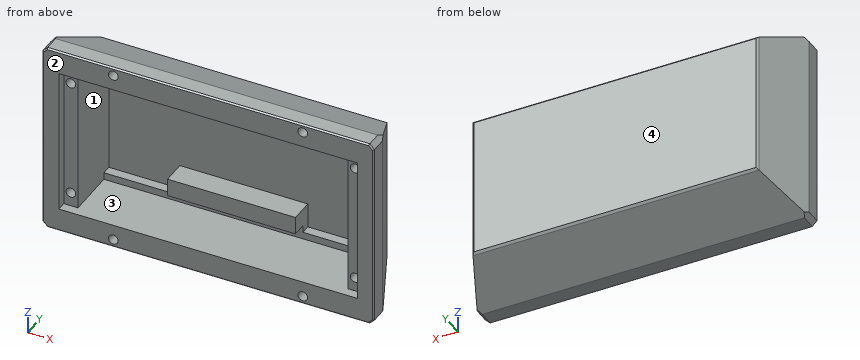
```python
from build123d import *
from OCP.BRepFilletAPI import BRepFilletAPI_MakeChamfer

# Parameters (mm, degrees)
SKETCH1_W                       = 140
SKETCH1_H                       = 82
BOSS_EXTRUDE1_DEPTH             = 7
SKETCH3_W                       = 140
SKETCH3_H                       = 82
SKETCH2_W                       = 120
SKETCH2_H                       = 60
CHAMFER1_SIZE                   = 2
SKETCH4_R                       = 2.05
CUT_EXTRUDE1_DEPTH              = 7
SKETCH5_W                       = 114
SKETCH5_H                       = 50
CUT_EXTRUDE2_DEPTH              = 29
SKETCH6_W                       = 114
SKETCH6_H                       = 62
CUT_EXTRUDE3_DEPTH              = 25
SKETCH7_W                       = 6
SKETCH7_H                       = 62
CUT_EXTRUDE4_DEPTH              = 4
SKETCH8_R                       = 2.05
CUT_EXTRUDE5_DEPTH              = 6
CHAMFER2_SIZE                   = 1
CHAMFER2_SIZE2                  = 0.471497246
CHAMFER2_SIZE2_2                = 0.488486876
CHAMFER3_SIZE                   = 0.6
SKIZZE1_W                       = 54.050484576
SKIZZE1_H                       = 7.5
SKIZZE1_W_2                     = 4
SKIZZE1_H_2                     = 21.453027382
AUFSATZ_LINEAR_AUSTRAGEN1_DEPTH = 10
SKIZZE3_W                       = 29.974757712
SKIZZE3_H                       = 3
SCHNITT_LINEAR_AUSTRAGEN2_DEPTH = 4


with BuildPart() as part:
    # Sketch1 → Boss-Extrude1 (new body)
    with BuildSketch(Plane(origin=(0, 0, 0), x_dir=(1, 0, 0), z_dir=(0, 1, 0))):
        Rectangle(SKETCH1_W, SKETCH1_H)
    extrude(amount=BOSS_EXTRUDE1_DEPTH)

    # Sketch3 → Loft2 section 0
    with BuildSketch(Plane(origin=(0, 7, 0), x_dir=(1, 0, 0), z_dir=(0, 1, 0))):
        Rectangle(SKETCH3_W, SKETCH3_H)
    # Sketch2 → Loft2 section 1
    with BuildSketch(Plane(origin=(0, 30, 0), x_dir=(1, 0, 0), z_dir=(0, 1, 0))):
        Rectangle(SKETCH2_W, SKETCH2_H)
    loft()

    # Chamfer1
    chamfer1_edges = [part.edges().sort_by_distance(p)[0] for p in [
        (-70, 3.5, 41),
        (70, 3.5, 41),
        (70, 3.5, -41),
        (-70, 3.5, -41),
    ]]
    chamfer(chamfer1_edges, length=CHAMFER1_SIZE)

    # Sketch4 → Cut-Extrude1 (cut)
    with BuildSketch(Plane.XZ):
        with Locations(Location((40, -37.5, 0), (0, 0, 270))):
            Circle(SKETCH4_R)
        with Locations(Location((-40, -37.5, 0), (0, 0, 270))):
            Circle(SKETCH4_R)
    cut_extrude1 = extrude(amount=-CUT_EXTRUDE1_DEPTH, mode=Mode.SUBTRACT)

    # Sketch5 → Cut-Extrude2 (cut)
    with BuildSketch(Plane.XZ):
        Rectangle(SKETCH5_W, SKETCH5_H)
    extrude(amount=-CUT_EXTRUDE2_DEPTH, mode=Mode.SUBTRACT)

    # Mirror1: Cut-Extrude1 across plane
    add(cut_extrude1.mirror(Plane.XY), mode=Mode.SUBTRACT)

    # Sketch6 → Cut-Extrude3 (cut)
    with BuildSketch(Plane.XZ):
        Rectangle(SKETCH6_W, SKETCH6_H)
    extrude(amount=-CUT_EXTRUDE3_DEPTH, mode=Mode.SUBTRACT)

    # Sketch7 → Cut-Extrude4 (cut)
    with BuildSketch(Plane.XZ):
        with Locations((-60, 0)):
            Rectangle(SKETCH7_W, SKETCH7_H)
        with Locations((60, 0)):
            Rectangle(SKETCH7_W, SKETCH7_H)
    extrude(amount=-CUT_EXTRUDE4_DEPTH, mode=Mode.SUBTRACT)

    # Sketch8 → Cut-Extrude5 (cut)
    with BuildSketch(Plane.XZ.offset(-4)):
        with Locations(Location((-60, 25, 0), (0, 0, 270))):
            Circle(SKETCH8_R)
        with Locations(Location((-60, -25, 0), (0, 0, 270))):
            Circle(SKETCH8_R)
        with Locations(Location((60, -25, 0), (0, 0, 90))):
            Circle(SKETCH8_R)
        with Locations(Location((60, 25, 0), (0, 0, 90))):
            Circle(SKETCH8_R)
    extrude(amount=-CUT_EXTRUDE5_DEPTH, mode=Mode.SUBTRACT)

    # Chamfer2: one chamfer whose edges measure the first distance from different faces: ONE call of the kernel's chamfer builder (chamfer() names one face for all edges)
    chamfer2_edges_1 = [part.edges().sort_by_distance(p)[0] for p in [
        (60, 30, 0),
    ]]
    chamfer2_side_1 = [part.faces().sort_by_distance(p)[0] for p in [
        (65.246314621, 17.933476372, 0),
    ]]
    chamfer2_edges_2 = [part.edges().sort_by_distance(p)[0] for p in [
        (0, 30, -30),
    ]]
    chamfer2_side_2 = [part.faces().sort_by_distance(p)[0] for p in [
        (0, 18.220498667, -35.633674551),
    ]]
    chamfer2_edges_3 = [part.edges().sort_by_distance(p)[0] for p in [
        (-60, 30, 0),
    ]]
    chamfer2_side_3 = [part.faces().sort_by_distance(p)[0] for p in [
        (-65.246314621, 17.933476372, 0),
    ]]
    chamfer2_edges_4 = [part.edges().sort_by_distance(p)[0] for p in [
        (0, 30, 30),
    ]]
    chamfer2_side_4 = [part.faces().sort_by_distance(p)[0] for p in [
        (0, 18.220498667, 35.633674551),
    ]]
    chamfer2 = BRepFilletAPI_MakeChamfer(part.part.solid().wrapped)
    for e in chamfer2_edges_1:
        chamfer2.Add(CHAMFER2_SIZE, CHAMFER2_SIZE2, e.wrapped, chamfer2_side_1[0].wrapped)  # the first distance lies on this face
    for e in chamfer2_edges_2:
        chamfer2.Add(CHAMFER2_SIZE, CHAMFER2_SIZE2_2, e.wrapped, chamfer2_side_2[0].wrapped)  # the first distance lies on this face
    for e in chamfer2_edges_3:
        chamfer2.Add(CHAMFER2_SIZE, CHAMFER2_SIZE2, e.wrapped, chamfer2_side_3[0].wrapped)  # the first distance lies on this face
    for e in chamfer2_edges_4:
        chamfer2.Add(CHAMFER2_SIZE, CHAMFER2_SIZE2_2, e.wrapped, chamfer2_side_4[0].wrapped)  # the first distance lies on this face
    add(Compound.cast(chamfer2.Shape()), mode=Mode.REPLACE)

    # Chamfer3
    chamfer3_edges = [part.edges().sort_by_distance(p)[0] for p in [
        (0, 0, 41),
        (70, 0, 0),
        (-70, 0, 0),
        (0, 0, -41),
        (-69, 0, -40),
        (69, 0, -40),
        (69, 0, 40),
        (-69, 0, 40),
    ]]
    chamfer(chamfer3_edges, length=CHAMFER3_SIZE)

    # Skizze1 → Aufsatz-Linear austragen1 (add)
    with BuildSketch(Plane.XZ.offset(-29)):
        with Locations((0, -21.25)):
            Rectangle(SKIZZE1_W, SKIZZE1_H)
        with Locations((0, 21.25)):
            Rectangle(SKIZZE1_W, SKIZZE1_H)
        with Locations((55, 0)):
            Rectangle(SKIZZE1_W_2, SKIZZE1_H_2)
    extrude(amount=AUFSATZ_LINEAR_AUSTRAGEN1_DEPTH)

    # Skizze3 → Schnitt-Linear austragen2 (cut)
    with BuildSketch(Plane(origin=(0, 29, 0), x_dir=(-1, 0, 0), z_dir=(0, -1, 0))):
        with Locations((42.012621144, -26.5)):
            Rectangle(SKIZZE3_W, SKIZZE3_H)
        with Locations((-42.012621144, -26.5)):
            Rectangle(SKIZZE3_W, SKIZZE3_H)
        with Locations((42.012621144, 26.5)):
            Rectangle(SKIZZE3_W, SKIZZE3_H)
        with Locations((-42.012621144, 26.5)):
            Rectangle(SKIZZE3_W, SKIZZE3_H)
    extrude(amount=SCHNITT_LINEAR_AUSTRAGEN2_DEPTH, mode=Mode.SUBTRACT)


solid = part.part
```
Check sheet for the modelled part. Datum: model origin and axes. Units: mm. Face numbers are marked on the shaded views. A direction names the side the tool comes from. Round coordinates to 2 decimals unless told otherwise and drop trailing zeros. Write item = value, one per line.
Q1. Tool access check on the marked faces 3 and 4. Record the directions out of +Z, -Z, +X, -X, +Y, -Y that give a thin tool (end or side, any length) a straight path to the whole face; none if there is none.
Computed:
face_3 = -Y
face_4 = +Z, -Z, +X, -X, +Y
Q2. Draft check along Z on the marked faces 1 and 2. Enter one of: pulls with the +Z half, pulls with the -Z half, needs draft (parallel to the pull), parting line crosses it, or undercut.
Computed:
face_1 = undercut
face_2 = needs draft
Q3. Go/stop test with flat-tipped pins: pin 1 (5 mm diameter, centred on x = 36, y = 14, fed in from +Z); pin 2 (8 mm diameter, centred on y = 22, z = -24.5, fed in from +X); pin 3 (4.5 mm diameter, centred on x = 54, y = 21.5, fed in from -Z). Record where each tip stops, or that it passes through.
Computed:
pin_1 = 38.85
pin_2 = 65.22
pin_3 = -35.14
Q4. Thickness scan on line 1 along X through (y, z) = (5.5, 37.5); line 2 along Z through (x, y) = (-52.5, 3); line 3 along X through (y, z) = (5, -15.5). Record the ranges inside material, lowest first.
Computed:
line_1 = -70 to -42.05, -37.95 to 37.95, 42.05 to 70
line_2 = -41 to -31, 31 to 41
line_3 = -70 to -57, 57 to 70
